Design review of the part built by this model. Coordinates are the model's own, in mm. A direction names the side the tool comes from. Round coordinates to 2 decimals unless told otherwise and drop trailing zeros. Order: outer loops, then holes, each group sorted by start corner. A loop starts at its lowest first (then second) coordinate and runs counter-clockwise, first axis right, second up.
from build123d import *

# Parameters (mm, degrees)
SKETCH1_W           = 116
SKETCH1_H           = 61
SKETCH1_W_2         = 110
SKETCH1_H_2         = 55
BOSS_EXTRUDE1_DEPTH = 60
SKETCH2_W           = 116
SKETCH2_H           = 61
BOSS_EXTRUDE2_DEPTH = 3
CHAMFER1_SIZE       = 5
CHAMFER2_SIZE       = 6
SKETCH3_R           = 1.55
CUT_EXTRUDE1_DEPTH  = 3
SKETCH4_W           = 10
SKETCH4_H           = 15
CUT_EXTRUDE2_DEPTH  = 3
SKETCH5_R           = 1.4
CUT_EXTRUDE3_DEPTH  = 20
FILLET1_R           = 2
CHAMFER3_SIZE       = 12
CHAMFER4_SIZE       = 10
SKETCH6_W           = 58.5
SKETCH6_H           = 9.5
CUT_EXTRUDE4_DEPTH  = 10
SKETCH7_R           = 1.4
CUT_EXTRUDE5_DEPTH  = 10
SKETCH8_R           = 3
SKETCH8_R_2         = 1.4
BOSS_EXTRUDE3_DEPTH = 4


with BuildPart() as part:
    # Sketch1 → Boss-Extrude1 (new body)
    with BuildSketch(Plane(origin=(0, 0, 0), x_dir=(1, 0, 0), z_dir=(0, 1, 0))):
        Rectangle(SKETCH1_W, SKETCH1_H)
        Rectangle(SKETCH1_W_2, SKETCH1_H_2, mode=Mode.SUBTRACT)
    extrude(amount=BOSS_EXTRUDE1_DEPTH)

    # Sketch2 → Boss-Extrude2 (add)
    with BuildSketch(Plane(origin=(0, 60, 0), x_dir=(1, 0, 0), z_dir=(0, 1, 0))):
        Rectangle(SKETCH2_W, SKETCH2_H)
    extrude(amount=BOSS_EXTRUDE2_DEPTH)

    # Chamfer1
    chamfer1_edges = [part.edges().sort_by_distance(p)[0] for p in [
        (58, 31.5, 30.5),
        (-58, 31.5, 30.5),
        (-58, 31.5, -30.5),
        (58, 31.5, -30.5),
    ]]
    chamfer(chamfer1_edges, length=CHAMFER1_SIZE)

    # Chamfer2
    chamfer2_edges = [part.edges().sort_by_distance(p)[0] for p in [
        (55, 30, 27.5),
        (55, 30, -27.5),
        (-55, 30, -27.5),
        (-55, 30, 27.5),
    ]]
    chamfer(chamfer2_edges, length=CHAMFER2_SIZE)

    # Sketch3 → Cut-Extrude1 (cut)
    with BuildSketch(Plane(origin=(0, 63, 0), x_dir=(1, 0, 0), z_dir=(0, 1, 0))):
        with Locations(Location((30, 0, 0), (0, 0, 270))):
            Circle(SKETCH3_R)
        with Locations(Location((-30, 0, 0), (0, 0, 270))):
            Circle(SKETCH3_R)
    extrude(amount=-CUT_EXTRUDE1_DEPTH, mode=Mode.SUBTRACT)

    # Sketch4 → Cut-Extrude2 (cut)
    with BuildSketch(Plane(origin=(0, 63, 0), x_dir=(1, 0, 0), z_dir=(0, 1, 0))):
        with Locations((-8, 0.5)):
            Rectangle(SKETCH4_W, SKETCH4_H)
    extrude(amount=-CUT_EXTRUDE2_DEPTH, mode=Mode.SUBTRACT)

    # Sketch5 → Cut-Extrude3 (cut)
    with BuildSketch(Plane.XZ):
        with Locations(Location((53.7, -26.2, 0), (0, 0, 270))):
            Circle(SKETCH5_R)
        with Locations(Location((-53.7, -26.2, 0), (0, 0, 270))):
            Circle(SKETCH5_R)
        with Locations(Location((-53.7, 26.2, 0), (0, 0, 270))):
            Circle(SKETCH5_R)
        with Locations(Location((53.7, 26.2, 0), (0, 0, 270))):
            Circle(SKETCH5_R)
    extrude(amount=-CUT_EXTRUDE3_DEPTH, mode=Mode.SUBTRACT)

    # Fillet1
    fillet1_edges = [part.edges().sort_by_distance(p)[0] for p in [
        (-3, 61.5, -8),
        (-3, 61.5, 7),
        (-13, 61.5, 7),
        (-13, 61.5, -8),
    ]]
    fillet(fillet1_edges, radius=FILLET1_R)

    # Chamfer3
    chamfer3_edges = [part.edges().sort_by_distance(p)[0] for p in [
        (58, 63, 0),
        (-58, 63, 0),
    ]]
    chamfer(chamfer3_edges, length=CHAMFER3_SIZE)

    # Chamfer4
    chamfer4_edges = [part.edges().sort_by_distance(p)[0] for p in [
        (55, 60, 0),
        (-55, 60, 0),
    ]]
    chamfer(chamfer4_edges, length=CHAMFER4_SIZE)

    # Sketch6 → Cut-Extrude4 (cut)
    with BuildSketch(Plane(origin=(0, 0, -30.5), x_dir=(-1, 0, 0), z_dir=(0, 0, -1))):
        with Locations((0, 4.75)):
            Rectangle(SKETCH6_W, SKETCH6_H)
    extrude(amount=-CUT_EXTRUDE4_DEPTH, mode=Mode.SUBTRACT)

    # Sketch7 → Cut-Extrude5 (cut)
    with BuildSketch(Plane(origin=(0, 63, 0), x_dir=(1, 0, 0), z_dir=(0, 1, 0))):
        with Locations(Location((7.959772519, 0, 0), (0, 0, 270))):
            Circle(SKETCH7_R)
        with Locations(Location((17.959772519, 0, 0), (0, 0, 270))):
            Circle(SKETCH7_R)
    extrude(amount=-CUT_EXTRUDE5_DEPTH, mode=Mode.SUBTRACT)

    # Sketch8 → Boss-Extrude3 (add)
    # profile 1 of 2: a face of its own
    with BuildSketch(Plane.XZ.offset(-60)):
        with Locations(Location((7.959772519, 0, 0), (0, 0, 90))):
            Circle(SKETCH8_R)
        with Locations(Location((7.959772519, 0, 0), (0, 0, 90))):
            Circle(SKETCH8_R_2, mode=Mode.SUBTRACT)
    # profile 2 of 2: a face of its own
    with BuildSketch(Plane.XZ.offset(-60)):
        with Locations(Location((17.959772519, 0, 0), (0, 0, 90))):
            Circle(SKETCH8_R)
        with Locations(Location((17.959772519, 0, 0), (0, 0, 90))):
            Circle(SKETCH8_R_2, mode=Mode.SUBTRACT)
    extrude(amount=BOSS_EXTRUDE3_DEPTH)


solid = part.part
1) To check wall thickness, follow line 1 along X through (y, z) = (40, -20); line 2 along Z through (x, y) = (30, 16); line 3 along X through (y, z) = (13, 26). State the ranges of each line that lie inside material, in increasing order.
Results:
line 1: x = -58 to -55, 55 to 58
line 2: z = -30.5 to -27.5, 27.5 to 30.5
line 3: x = -57.5 to -55.09, -52.31 to -50.5, 50.5 to 52.31, 55.09 to 57.5
2) Take a section at C-C on x = 26. Give the boundary of the cut face in (y, z), plus the area to 4 significant figures.
Results:
outline: (0, 27.5) - (60, 27.5) - (60, -27.5) - (9.5, -27.5) - (9.5, -30.5) - (63, -30.5) - (63, 30.5) - (0, 30.5) - close
area: 514.5 mm2
3) Take a section at D-D on y = 53. Give the boundary of the cut face in (x, z).
Results:
outline: (-56, -27.5) - (-53, -30.5) - (53, -30.5) - (56, -27.5) - (56, 27.5) - (53, 30.5) - (-53, 30.5) - (-56, 27.5) - close; hole (-52, -24.5) - (-49, -27.5) - (49, -27.5) - (52, -24.5) - (52, 24.5) - (49, 27.5) - (-49, 27.5) - (-52, 24.5) - close
4) The part is to be moulded in two halves that separate along Z. For faces 1 (the face through (55.5, 28.4, -28)), 2 (the face through (-29.25, 5, -29)), 3 (the face through (-55.067, 9.86, -25.897)), 4 (the face through (55, 25, 0)), say which applies: released by +Z, released by -Z, zero draft, split by the parting line, or undercut.
Results:
face 1: released by -Z
face 2: zero draft
face 3: undercut
face 4: undercut
5) Take a section at B-B on z = 16. Give the boundary of the cut face in (x, y).
Results:
outline: (-58, 0) - (-55, 0) - (-55, 50) - (-45, 60) - (45, 60) - (55, 50) - (55, 0) - (58, 0) - (58, 51) - (46, 63) - (-46, 63) - (-58, 51) - close
6) For faces 5 (the face through (0, 9.5, -29)), 6 (the face through (-3, 62, 0)), 7 (the face through (-54, 20, -26)), list the 3-axis set-ups (+Z, -Z, +X, -X, +Y, -Y) from which the entire face can be reached by the end or side of a thin tool; tool diameter is ignored.
Results:
face 5: -Z, -Y
face 6: +Y, -Y
face 7: -Y
7) Take a section at A-A on y = 11.5. Give the boundary of the cut face in (x, z), plus the area to 3 significant figures.
Results:
outline: (-58, -25.5) - (-53, -30.5) - (53, -30.5) - (58, -25.5) - (58, 25.5) - (53, 30.5) - (-53, 30.5) - (-58, 25.5) - close; hole circle Ø2.8 at (-53.7, -26.2); hole circle Ø2.8 at (-53.7, 26.2); hole (-55, -21.5) - (-49, -27.5) - (49, -27.5) - (55, -21.5) - (55, 21.5) - (49, 27.5) - (-49, 27.5) - (-55, 21.5) - close; hole circle Ø2.8 at (53.7, -26.2); hole circle Ø2.8 at (53.7, 26.2)
area: 1,020 mm2
8) Clearance check with flat-ended pins moving along their axes: P1, Ø10, axis at x = -10, z = -3.5, coming from the -Y side; P2, Ø2.5, axis at x = -53.7, z = -26.2, coming from the +Y side; P3, Ø3.5, axis at y = 3.5, z = -29, coming from the +X side. State where each tip first meets the part, or that it passes through.
Results:
P1: stops at y = 60
P2: stops at y = 56.55
P3: stops at x = 56.25
